Job drawing, mm, ordinate dimensions from the low corner. One solid piece. A direction names the side the tool comes from. Coordinates: 2 decimals unless noted, no trailing zeros. Order: outer loops, then holes, each group sorted by start corner. A loop starts at its lowest first (then second) coordinate and runs counter-clockwise, first axis right, second up. Notation, with made-up numbers: (-25, 62.25) - (-20, 62.25) arc R14 ccw to (-20, 70.25) - close; hole circle Ø10 at (60.5, -31.75). An arc over 180 degrees is marked (long way). Use one line per item in the form item = value.
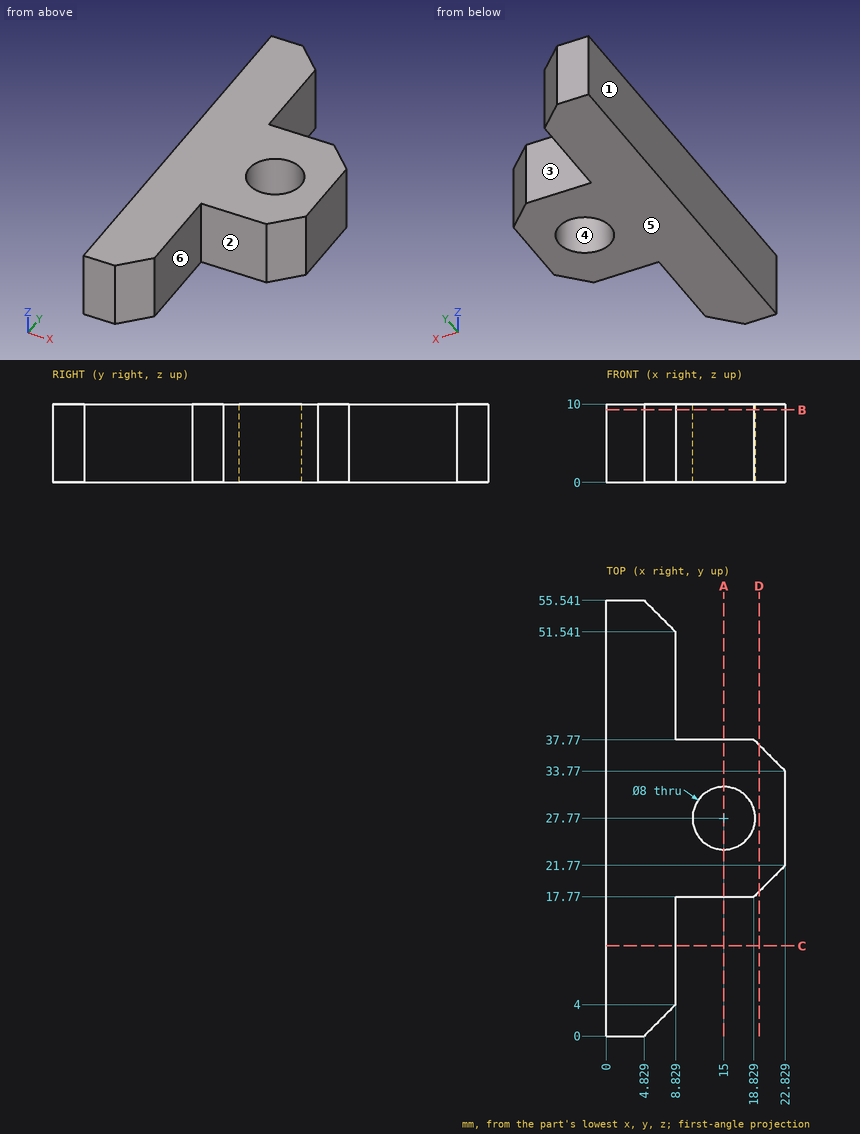
Item 1: Drill centre lines: line 1 (X direction, y = 17, z = 7); line 2 (Y direction, x = 15, z = 4); line 3 (X direction, y = 27.5, z = 0.75). Where is each one in solid material? Low to high. Write a range as [from, to].
Derived:
line_1 = [0, 8.83]
line_2 = [17.77, 23.77], [31.77, 37.77]
line_3 = [0, 11.01], [18.99, 22.83]
Item 2: Two-plate mould, pull along X, no slides. Class the marked faces 4, 5 and 6: +X half, -X half, draft (parallel to the pull), parting line (faces both ways), or undercut.
Derived:
face_4 = undercut
face_5 = draft
face_6 = +X half
Item 3: 3-axis set-ups, long thin cutter, end or side, ignore diameter. For the marked faces 1, 2 and 3: which of +Z, -Z, +X, -X, +Y, -Y reach the whole face in a straight line?
Derived:
face_1 = +Z, -Z, -X, +Y, -Y
face_2 = +Z, -Z, +X, -Y
face_3 = +Z, -Z, +X, +Y
Item 4: Cut at C-C, the plane y = 11.5. Write the cut outline in (x, z), plus the area to 3 significant figures.
Derived:
outline = (0, 0) - (8.83, 0) - (8.83, 10) - (0, 10) - close
area = 88.3 mm²
Item 5: Cut at B-B, the plane z = 9.25. Write the cut outline in (x, y).
Derived:
outline = (0, 0) - (4.83, 0) - (8.83, 4) - (8.83, 17.77) - (18.83, 17.77) - (22.83, 21.77) - (22.83, 33.77) - (18.83, 37.77) - (8.83, 37.77) - (8.83, 51.54) - (4.83, 55.54) - (0, 55.54) - close; hole circle Ø8 at (15, 27.77)
Item 6: Cut at D-D, the plane x = 19.5. Write the cut outline in (y, z), plus the area to 3 significant figures.
Derived:
outline = (18.44, 0) - (37.1, 0) - (37.1, 10) - (18.44, 10) - close
area = 187 mm²
Item 7: Cut at A-A, the plane x = 15. Write the cut outline in (y, z).
Derived:
outline = (17.77, 0) - (23.77, 0) - (23.77, 10) - (17.77, 10) - close; (31.77, 0) - (37.77, 0) - (37.77, 10) - (31.77, 10) - close
Item 8: Drop flat-ended pins along their axis: pin 1 (3 mm diameter, centred on y = 13.5, z = 3, fed in from +X); pin 2 (6 mm diameter, centred on x = 19, z = 8, fed in from -Y). Give the stop position or say it passes through.
Derived:
pin_1 = 8.83
pin_2 = 17.77
